Verification items for the finished model (mm, model axes). A direction names the side the tool comes from. Round coordinates to 2 decimals unless told otherwise and drop trailing zeros. Order: outer loops, then holes, each group sorted by start corner. A loop starts at its lowest first (then second) coordinate and runs counter-clockwise, first axis right, second up. Notation, with made-up numbers: (59.25, 48.25) -> (96.25, 48.25) arc R11 ccw to (96.25, 63.25) -> close; hole circle Ø1 at (43, -31.5). An arc over 180 degrees is marked (long way). Return JSON: item names as keys, results as strings. Group by question number.
Item 1: Draft check along Y on faces 4 (the flat face through (42.3, 7, 18.1)), 5 (the cylindrical face through (-43.836, 7.992, -21.306)), 6 (the cylindrical face through (20.94, 1.27, 21.66)). Enter one of: pulls with the +Y half, pulls with the -Y half, needs draft (parallel to the pull), parting line crosses it, or undercut.
Item 2: Sectioned sample at D-D on z = 41.5. Record the cut outline in (x, y).
Item 3: Sectioned sample at C-C on z = -7.5. Record the cut outline in (x, y).
Item 4: Scan lines: probe 1 along X at (y, z) = (3.5, -17); probe 2 along Z at (x, y) = (0, 2.65); probe 3 along X at (y, z) = (1.9, 7.5). Record each from-to range of solid material in increasing order. Write a range as from..to.
Item 5: Access from +Z, -Z, +X, -X, +Y, -Y to the whole of each face (thin tool, end or side, straight path). Record for faces 1 (the cylindrical face through (-20.847, 1.479, 7.37)), 2 (the flat face through (42.794, 11.311, 20.622)), 3 (the flat face through (30.784, 10.541, -28.613)).
Item 6: Sectioned sample at A-A on y = 13.25. Give the number of separate pieces and of enclosed holes in the cut face, plus the area to 3 significant figures.
Item 7: Depth check by flat-ended pin: pin 1 Ø1 at (y, z) = (7, 35) entering from -X; pin 2 Ø4 at (y, z) = (9.5, 15) entering from -X; pin 3 Ø1.7 at (x, z) = (21, -21) entering from +Y. Enter the tip coordinate at first touch or a pass-through.
Item 8: Sectioned sample at B-B on x = 0. Record the cut outline in (y, z), plus the area to 3 significant figures.
```python
from build123d import *

# Parameters (mm, degrees)
CROQUIS1_W               = 43
CROQUIS1_H               = 4.5
CROQUIS2_R               = 1.7
CORTAR_EXTRUIR1_DEPTH    = 10
CORTAR_EXTRUIR2_DEPTH    = 2
CROQUIS4_R               = 2.95
CORTAR_EXTRUIR3_DEPTH    = 3
SALIENTE_EXTRUIR1_DEPTH  = 10
CROQUIS6_R               = 1.7
CORTAR_EXTRUIR4_DEPTH    = 10
CORTAR_EXTRUIR5_DEPTH    = 1.5
MATRIZC1_COUNT           = 2
MATRIZC1_ANGLE           = 70
MATRIZC2_COUNT           = 2
MATRIZC2_COPY_1_DEPTH    = 10
MATRIZC2_COPY_2_SKETCH_R = 1.7
MATRIZC2_COPY_2_DEPTH    = 10
MATRIZC2_COPY_3_DEPTH    = 1.5


with BuildPart() as part:
    # Croquis1 → Revoluci_n1 (revolve)
    with BuildSketch(Plane.XY):
        with Locations((33.5, 2.25)):
            Rectangle(CROQUIS1_W, CROQUIS1_H)
    revolve(axis=Axis((0, 115.94715176, 0), (0, -1, 0)))

    # Croquis2 → Cortar-Extruir1 (cut)
    with BuildSketch(Plane(origin=(0, 4.5, 0), x_dir=(1, 0, 0), z_dir=(0, 1, 0))):
        with Locations((-31.7, 7.5)):
            Circle(CROQUIS2_R)
        with Locations((17.9, 7.5)):
            Circle(CROQUIS2_R)
        with Locations((-17.9, -7.5)):
            Circle(CROQUIS2_R)
        with Locations((31.7, -7.5)):
            Circle(CROQUIS2_R)
        with Locations((20.152543264, 20.152543264)):
            Circle(CROQUIS2_R)
        with Locations((-20.152543264, 20.152543264)):
            Circle(CROQUIS2_R)
        with Locations((-20.152543264, -20.152543264)):
            Circle(CROQUIS2_R)
        with Locations((20.152543264, -20.152543264)):
            Circle(CROQUIS2_R)
    extrude(amount=-CORTAR_EXTRUIR1_DEPTH, mode=Mode.SUBTRACT)

    # Croquis3 → Cortar-Extruir2 (cut)
    with BuildSketch(Plane(origin=(0, 4.5, 0), x_dir=(1, 0, 0), z_dir=(0, 1, 0))):
        Polygon((-20.152543264, 23.502543264), (-23.053728366, 21.827543264), (-23.053728366, 18.477543264), (-20.152543264, 16.802543264), (-17.251358161, 18.477543264), (-17.251358161, 21.827543264), align=None)
        Polygon((20.152543264, 23.502543264), (17.251358161, 21.827543264), (17.251358161, 18.477543264), (20.152543264, 16.802543264), (23.053728366, 18.477543264), (23.053728366, 21.827543264), align=None)
        Polygon((-20.152543264, -16.802543264), (-23.053728366, -18.477543264), (-23.053728366, -21.827543264), (-20.152543264, -23.502543264), (-17.251358161, -21.827543264), (-17.251358161, -18.477543264), align=None)
        Polygon((20.152543264, -16.802543264), (17.251358161, -18.477543264), (17.251358161, -21.827543264), (20.152543264, -23.502543264), (23.053728366, -21.827543264), (23.053728366, -18.477543264), align=None)
    extrude(amount=-CORTAR_EXTRUIR2_DEPTH, mode=Mode.SUBTRACT)

    # Croquis4 → Cortar-Extruir3 (cut)
    with BuildSketch(Plane(origin=(0, 0, 0), x_dir=(1, 0, 0), z_dir=(0, 1, 0))):
        with Locations((-31.7, 7.5)):
            Circle(CROQUIS4_R)
        with Locations((-17.9, -7.5)):
            Circle(CROQUIS4_R)
        with Locations((17.9, 7.5)):
            Circle(CROQUIS4_R)
        with Locations((31.7, -7.5)):
            Circle(CROQUIS4_R)
    extrude(amount=CORTAR_EXTRUIR3_DEPTH, mode=Mode.SUBTRACT)

    # Croquis5 → Saliente-Extruir1 (add)
    with BuildSketch(Plane(origin=(0, 4.5, 0), x_dir=(1, 0, 0), z_dir=(0, 1, 0))):
        with BuildLine():
            Line((-34.294678888, -25.102290732), (-25.102290732, -34.294678888))
            Line((-25.102290732, -34.294678888), (-30.459119357, -39.651507512))
            ThreePointArc((-30.459119357, -39.651507512), (-35.355339059, -35.355339059), (-39.651507512, -30.459119357))
            Line((-39.651507512, -30.459119357), (-34.294678888, -25.102290732))
        make_face()
    saliente_extruir1 = extrude(amount=SALIENTE_EXTRUIR1_DEPTH)

    # Croquis6 → Cortar-Extruir4 (cut)
    with BuildSketch(Plane(origin=(-29.69848481, 0, 29.69848481), x_dir=(-0.707106781, 0, -0.707106781), z_dir=(0.707106781, 0, -0.707106781))):
        with Locations((0, 9.5)):
            Circle(CROQUIS6_R)
    cortar_extruir4 = extrude(amount=-CORTAR_EXTRUIR4_DEPTH, mode=Mode.SUBTRACT)

    # Croquis7 → Cortar-Extruir5 (cut, symmetric)
    with BuildSketch(Plane(origin=(-32.526911935, 0, 32.526911935), x_dir=(0.707106781, 0, 0.707106781), z_dir=(-0.707106781, 0, 0.707106781))):
        Polygon((-2.901185103, 11.175), (-2.901185103, 17.825), (2.901185103, 17.825), (2.901185103, 11.175), (2.901185103, 7.825), (0, 6.15), (-2.901185103, 7.825), align=None)
    cortar_extruir5 = extrude(amount=CORTAR_EXTRUIR5_DEPTH, both=True, mode=Mode.SUBTRACT)

    # MatrizC1: Saliente-Extruir1, Cortar-Extruir4, Cortar-Extruir5 ×2 about axis
    matrizc1_axis = Axis((0, 0, 0), (0, -1, 0))
    for i in range(1, MATRIZC1_COUNT):
        add(saliente_extruir1.rotate(matrizc1_axis, i * MATRIZC1_ANGLE / (MATRIZC1_COUNT - 1)))
        add(cortar_extruir4.rotate(matrizc1_axis, i * MATRIZC1_ANGLE / (MATRIZC1_COUNT - 1)), mode=Mode.SUBTRACT)
        add(cortar_extruir5.rotate(matrizc1_axis, i * MATRIZC1_ANGLE / (MATRIZC1_COUNT - 1)), mode=Mode.SUBTRACT)

    # MatrizC2: Saliente-Extruir1, Cortar-Extruir4, Cortar-Extruir5 ×2 about axis
    matrizc2_axis = Axis((0, 0, 0), (0, 1, 0))
    for i in range(1, MATRIZC2_COUNT):
        add(saliente_extruir1.rotate(matrizc2_axis, i * 360 / MATRIZC2_COUNT))
        add(cortar_extruir4.rotate(matrizc2_axis, i * 360 / MATRIZC2_COUNT), mode=Mode.SUBTRACT)
        add(cortar_extruir5.rotate(matrizc2_axis, i * 360 / MATRIZC2_COUNT), mode=Mode.SUBTRACT)

    # MatrizC2 copy 1 sketch → MatrizC2 copy 1 (add)
    with BuildSketch(Plane(origin=(0, 4.5, 0), x_dir=(-0.342020143, 0, -0.939692621), z_dir=(0, 1, 0))):
        with BuildLine():
            Line((-34.294678888, -25.102290732), (-25.102290732, -34.294678888))
            Line((-25.102290732, -34.294678888), (-30.459119357, -39.651507512))
            ThreePointArc((-30.459119357, -39.651507512), (-35.355339059, -35.355339059), (-39.651507512, -30.459119357))
            Line((-39.651507512, -30.459119357), (-34.294678888, -25.102290732))
        make_face()
    extrude(amount=MATRIZC2_COPY_1_DEPTH)

    # MatrizC2 copy 2 sketch → MatrizC2 copy 2 (cut)
    with BuildSketch(Plane(origin=(38.064927056, 0, 17.749966993), x_dir=(-0.422618262, 0, 0.906307787), z_dir=(-0.906307787, 0, -0.422618262))):
        with Locations((0, 9.5)):
            Circle(MATRIZC2_COPY_2_SKETCH_R)
    extrude(amount=-MATRIZC2_COPY_2_DEPTH, mode=Mode.SUBTRACT)

    # MatrizC2 copy 3 sketch → MatrizC2 copy 3 (cut, symmetric)
    with BuildSketch(Plane(origin=(41.690158204, 0, 19.44044004), x_dir=(0.422618262, 0, -0.906307787), z_dir=(0.906307787, 0, 0.422618262))):
        Polygon((-2.901185103, 11.175), (-2.901185103, 17.825), (2.901185103, 17.825), (2.901185103, 11.175), (2.901185103, 7.825), (0, 6.15), (-2.901185103, 7.825), align=None)
    extrude(amount=MATRIZC2_COPY_3_DEPTH, both=True, mode=Mode.SUBTRACT)


solid = part.part
```
Recorded:
{
 "1": {"face 4": "pulls with the +Y half", "face 5": "undercut", "face 6": "needs draft"},
 "2": {"outline": "(-36.09, 0) -> (36.09, 0) -> (36.09, 4.5) -> (-36.09, 4.5) -> close"},
 "3": {"outline": "(-54.49, 0) -> (-34.65, 0) -> (-34.65, 3) -> (-33.4, 3) -> (-33.4, 4.5) -> (-54.49, 4.5) -> close; (-30, 3) -> (-28.75, 3) -> (-28.75, 0) -> (-9.37, 0) -> (-9.37, 4.5) -> (-30, 4.5) -> close; (9.37, 0) -> (14.95, 0) -> (14.95, 3) -> (16.2, 3) -> (16.2, 4.5) -> (9.37, 4.5) -> close; (19.6, 3) -> (20.85, 3) -> (20.85, 0) -> (54.49, 0) -> (54.49, 4.5) -> (19.6, 4.5) -> close"},
 "4": {"probe 1": "-52.31..-20.49, -19.81..19.81, 20.49..52.31", "probe 2": "-55..-12, 12..55", "probe 3": "-54.49..-20.85, -14.95..-9.37, 9.37..28.75, 34.65..54.49"},
 "5": {"face 1": "-Y", "face 2": "+Y", "face 3": "+Z, +Y"},
 "6": {"separate pieces": "4", "enclosed holes": "4", "area": "339 mm²"},
 "7": {"pin 1": "x = -36.19", "pin 2": "x = 38.59", "pin 3": "y = 2.5"},
 "8": {"outline": "(0, -55) -> (4.5, -55) -> (4.5, -12) -> (0, -12) -> close; (0, 12) -> (4.5, 12) -> (4.5, 55) -> (0, 55) -> close", "area": "387 mm²"}
}
